Verification items for the finished model (mm, model axes). A direction names the side the tool comes from. Coordinates: 2 decimals unless noted, no trailing zeros. Order: outer loops, then holes, each group sorted by start corner. A loop starts at its lowest first (then second) coordinate and runs counter-clockwise, first axis right, second up.
Q1. Depth check by flat-ended pin: P1, Ø5, axis at x = -42.5, y = -0.5, coming from the +Z side; P2, Ø1, axis at x = 17, z = 44, coming from the +Y side; P3, Ø6, axis at x = 2, z = -2.5, coming from the +Y side; P4, Ø10, axis at x = -42.5, z = 17, coming from the +Y side. Enter the tip coordinate at first touch or a pass-through.
Q2. Cross-section at B-B, the plane y = 10.5. Record the boundary of the cut face in (x, z), and give its area (3 significant figures).
Q3. Thickness scan on line 1 (Y direction, x = -8.5, z = -5); line 2 (Z direction, x = 1, y = -3); line 3 (Y direction, x = -40, z = -35.5). Record the ranges inside material, lowest first.
Q4. Set-up check for faces 1 (the cylindrical face through (8.96, 11.81, -4.66)), 2 (the flat face through (0, 35, 0)): record each of +Z, -Z, +X, -X, +Y, -Y from which the full face is reachable in a straight line by a thin tool's end or side.
Q5. Cross-section at A-A, the plane y = 21.5. Record the boundary of the cut face in (x, z), and give its area (3 significant figures).
Q6. Draft check along Z on faces 3 (the cylindrical face through (7.81, 15.21, 1.73)), 4 (the flat face through (-1, -15, -1)), 5 (the cylindrical face through (79.845, -9.125, -41.53)), 6 (the flat face through (-8, 0, 3)). Enter one of: pulls with the +Z half, pulls with the -Z half, needs draft (parallel to the pull), parting line crosses it, or undercut.
from build123d import *


with BuildPart() as part:
    # 草图3 → 旋转1 (revolve)
    with BuildSketch(Plane.XY, mode=Mode.PRIVATE) as revolve_1_sk:
        with BuildLine():
            Line((90, -15), (90, -3.411628169))
            ThreePointArc((90, -3.411628169), (89.130160961, -0.593513474), (86.823291826, 1.24407875))
            Line((86.823291826, 1.24407875), (16.923291826, 28.61867531))
            ThreePointArc((16.923291826, 28.61867531), (12.281885305, 28.093129351), (10.1, 23.96296839))
            Line((10.1, 23.96296839), (10.1, 0))
            Line((10.1, 0), (8, 0))
            Line((8, 0), (8, 30))
            ThreePointArc((8, 30), (6.535533906, 33.535533906), (3, 35))
            Line((3, 35), (0, 35))
            Line((0, 35), (0, 0))
            Line((0, 0), (0, -15))
            Line((0, -15), (90, -15))
        make_face()
    revolve(revolve_1_sk.sketch.rotate(Axis((0, 0, 0), (0, 1, 0)), 90), axis=Axis((0, 0, 0), (0, 1, 0)))


solid = part.part
Check values:
1. P1: stops at z = 80.15
1. P2: stops at y = 16.97
1. P3: stops at y = 35
1. P4: stops at y = 19.28
2. outline: circle Ø126.38 at (0, 0); circle Ø16 at (0, 0); hole circle Ø20.2 at (0, 0)
2. area: 12,400 mm2
3. line 1: y = -15 to 0
3. line 2: z = -89.98 to 89.98
3. line 3: y = -15 to 14.3
4. face 1: +Y
4. face 2: +Z, -Z, +X, -X, +Y
5. outline: circle Ø70.2 at (0, 0); circle Ø16 at (0, 0); hole circle Ø20.2 at (0, 0)
5. area: 3,750 mm2
6. face 3: undercut
6. face 4: needs draft
6. face 5: parting line crosses it
6. face 6: undercut
